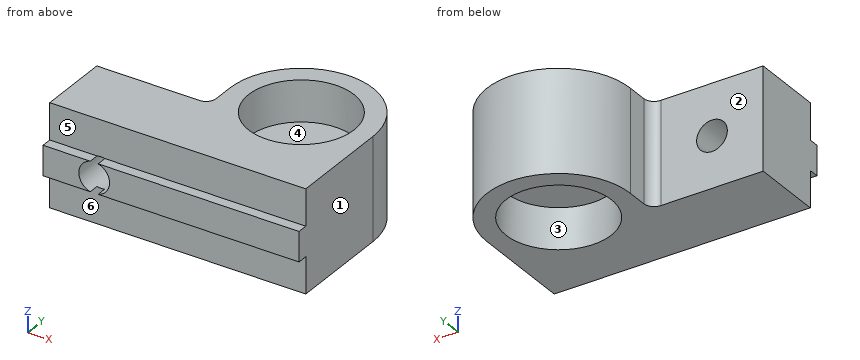
from build123d import *

# Parameters (mm, degrees)
SKETCH1_R              = 1.5
MAIN_DEPTH             = 5
SKETCH3_W              = 2.9
SKETCH3_H              = 1
MAKERBEAMRAIL_DEPTH    = 25
SKETCH2_R              = 1.5
MAKERBEAMFIXHOLE_DEPTH = 9
SKETCH4_R              = 5.15
ROLLINGHOLE_DEPTH      = 4
FILLET1_R              = 1


with BuildPart() as part:
    # Sketch1 → Main (new body, symmetric)
    with BuildSketch(Plane.XY):
        with BuildLine():
            Line((-18, 0), (7, 0))
            Line((7, 0), (7, 10))
            ThreePointArc((7, 10), (0, 17), (-7, 10))
            Line((-7, 10), (-7, 7))
            Line((-7, 7), (-18, 7))
            Line((-18, 7), (-18, 0))
        make_face()
        with Locations((0, 10)):
            Circle(SKETCH1_R, mode=Mode.SUBTRACT)
    extrude(amount=MAIN_DEPTH, both=True)

    # Sketch3 → MakerBeamRail (add)
    with BuildSketch(Plane.ZY.offset(18)):
        with Locations((0, -0.5)):
            Rectangle(SKETCH3_W, SKETCH3_H)
    extrude(amount=-MAKERBEAMRAIL_DEPTH)

    # Sketch2 → MakerBeamFixHole (cut, through all)
    with BuildSketch(Plane(origin=(0, 7, 0), x_dir=(1, 0, 0), z_dir=(0, 1, 0))):
        with Locations((-13, 0)):
            Circle(SKETCH2_R)
    extrude(amount=-MAKERBEAMFIXHOLE_DEPTH, mode=Mode.SUBTRACT)

    # Sketch4 → RollingHole (cut)
    with BuildSketch(Plane.XY.offset(5)):
        with Locations((0, 10)):
            Circle(SKETCH4_R)
    rollinghole = extrude(amount=-ROLLINGHOLE_DEPTH, mode=Mode.SUBTRACT)

    # MirrorRollingHole: RollingHole across plane
    add(rollinghole.mirror(Plane.XY), mode=Mode.SUBTRACT)

    # Fillet1
    fillet1_edges = [part.edges().sort_by_distance(p)[0] for p in [
        (-7, 7, 0),
    ]]
    fillet(fillet1_edges, radius=FILLET1_R)


solid = part.part
Read the model definition and answer for the solid it produces. Units are mm, in the model's axes. Face numbers are marked on the shaded views. A direction names the side the tool comes from. Round coordinates to 2 decimals unless told otherwise and drop trailing zeros. Write each loop counter-clockwise with the first axis right and the second up, starting at its lowest first coordinate (ties: lowest second). Pieces come first, ordered by that corner, then holes.
Q1. Straight lines are drawn through the part: line 1 (X direction, y = 4.5, z = 0); line 2 (Z direction, x = -13, y = 1); line 3 (X direction, y = 10, z = 0.1). For each, find the intervals that lie inside material, in ascending order.
Values:
line 1: x = -18 to -14.5, -11.5 to 7
line 2: z = -5 to -1.5, 1.5 to 5
line 3: x = -7 to -1.5, 1.5 to 7
Q2. The mould has two halves that part along X. Classify the marked faces 1, 2 and 3: released by +X, released by -X, zero draft, split by the parting line, or undercut.
Values:
face 1: released by +X
face 2: zero draft
face 3: undercut
Q3. Find section A-A on z = 0. Determine the outline of the cut face in (x, y).
Values:
outline: (-18, -1) - (-14.5, -1) - (-14.5, 7) - (-18, 7) - close; (-11.5, -1) - (7, -1) - (7, 10) arc R7 ccw to (-7, 10) - (-7, 8) arc R1 cw to (-8, 7) - (-11.5, 7) - close; hole circle Ø3 at (0, 10)
Q4. Find section C-C on z = 4.25. Determine the outline of the cut face in (x, y).
Values:
outline: (-18, 0) - (7, 0) - (7, 10) arc R7 ccw to (-7, 10) - (-7, 8) arc R1 cw to (-8, 7) - (-18, 7) - close; hole circle Ø10.3 at (0, 10)
Q5. Flat-ended cylindrical pins translate along their axes: P1, Ø2, axis at y = 9.5, z = -2, coming from the -X side; P2, Ø6, axis at x = 0, y = 10, coming from the -Z side; P3, Ø1.8, axis at x = -8, z = -3, coming from the -Y side; P4, Ø1, axis at x = -12.5, z = 0, coming from the -Y side. Find the tip coordinate at first contact, or state that the pin passes through.
Values:
P1: stops at x = -7
P2: stops at z = -1
P3: stops at y = 0
P4: passes through
Q6. Find section D-D on y = 1. Determine the outline of the cut face in (x, z), and give its area (3 significant figures).
Values:
outline: (-18, -5) - (7, -5) - (7, 5) - (-18, 5) - close; hole circle Ø3 at (-13, 0)
area: 243 mm2
Q7. Find section B-B on x = -13. Determine the outline of the cut face in (y, z), and give its area (3 significant figures).
Values:
outline: (0, -5) - (7, -5) - (7, -1.5) - (0, -1.5) - close; (0, 1.5) - (7, 1.5) - (7, 5) - (0, 5) - close
area: 49.0 mm2
Q8. A tool of negligible diameter and unlimited length cuts with its end or side. For the marked faces 4, 5 and 6, from which of +Z, -Z, +X, -X, +Y, -Y can it reach the whole face along a straight path? Write none if from no direction.
Values:
face 4: +Z
face 5: +Z, +X, -X, -Y
face 6: -Z, +X, -X, -Y
